Source: CAD feature listing. Evaluate the final solid. Frame: model axes, mm. Face numbers are marked on the shaded views. A direction names the side the tool comes from. Give positions to 0.01 mm unless a question says otherwise; leave off trailing zeros. Order: outer loops, then holes, each group sorted by start corner. A loop starts at its lowest first (then second) coordinate and runs counter-clockwise, first axis right, second up. Notation, with made-up numbers: (11.25, 44.25) - (51.25, 44.25) arc R32 ccw to (51.25, 73.25) - close; hole circle Ø7 at (61.25, -17.75). An arc over 180 degrees is marked (long way). Write each question's results on one line, items separated by ' | '. Start each with the question number.
Item 1: Section C-C on x = 67.5. Output: boundary loops of the cut face in (y, z), and give its area (3 significant figures).
Item 2: Section D-D on x = -80. Output: boundary loops of the cut face in (y, z).
Item 3: Section A-A on z = 45. Output: boundary loops of the cut face in (x, y), and give its area (3 significant figures).
Item 4: Contact query for flat-ended pins moving along their axis: pin 1 Ø4 at (y, z) = (-2.5, 62) entering from +X; pin 2 Ø8.5 at (x, y) = (26.5, 40) entering from +Z; pin 3 Ø8 at (x, y) = (-79.93, 17) entering from +Z; pin 4 Ø12 at (y, z) = (0, 45) entering from -X. Output: stop coordinate, or through.
Item 5: Mould query, pull axis Y, two halves, no side actions, for the marked faces 5, 6, 7 and 8. Classes: released by +Y, released by -Y, zero draft, split by the parting line, or undercut.
Item 6: Set-up query: the marked faces 1, 2, 3 and 4. Return all of +Z, -Z, +X, -X, +Y, -Y with unobstructed straight access to the full face (end or side cutting, diameter ignored); none if empty.
Item 7: Line query: line 1 along Y through (x, z) = (64, 45); line 2 along Y through (x, z) = (-80, 12.5); line 3 along Z through (x, y) = (-58, 9). Output: solid intervals per line, ascending.
Item 8: Section B-B on y = -17. Output: boundary loops of the cut face in (x, z).
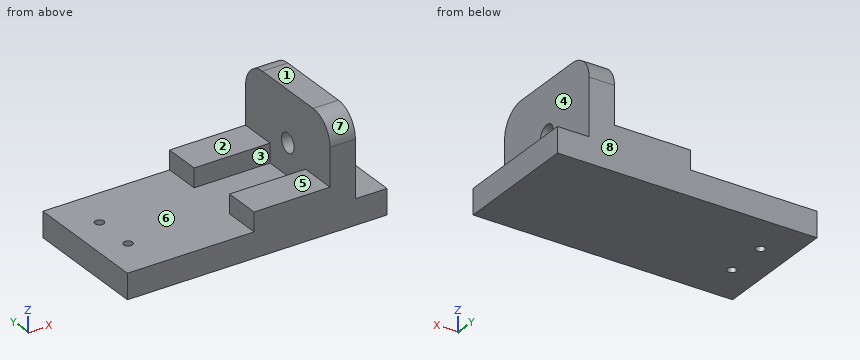
```python
from build123d import *

# Parameters (mm, degrees)
SCHIZZO1_W                   = 205
SCHIZZO1_H                   = 100
ESTRUSIONE_ESTRUSIONE1_DEPTH = 20
FORO_FILETTATO_M8X1_0_1_D    = 7
SCHIZZO6_W                   = 60
SCHIZZO6_H                   = 29
ESTRUSIONE_ESTRUSIONE2_DEPTH = 15
SCHIZZO7_W                   = 20
SCHIZZO7_H                   = 100
ESTRUSIONE_ESTRUSIONE3_DEPTH = 65
SCHIZZO8_R                   = 7.5
TAGLIO_ESTRUSIONE1_DEPTH     = 206.243757518
RACCORDO1_R                  = 20


with BuildPart() as part:
    # Schizzo1 → Estrusione-Estrusione1 (new body)
    with BuildSketch(Plane.XY):
        Rectangle(SCHIZZO1_W, SCHIZZO1_H)
    extrude(amount=ESTRUSIONE_ESTRUSIONE1_DEPTH)

    # Foro filettato M8x1.0-1 (through all)
    with Locations(Plane(origin=(0, 0, 0), x_dir=(-1, 0, 0), z_dir=(0, 0, -1))):
        with Locations((79.93168314, 16.999931365), (80, -17)):
            Hole(FORO_FILETTATO_M8X1_0_1_D / 2)

    # Schizzo6 → Estrusione-Estrusione2 (add)
    with BuildSketch(Plane.XY.offset(20)):
        with Locations((27.5, -35.5)):
            Rectangle(SCHIZZO6_W, SCHIZZO6_H)
        with Locations((27.5, 35.5)):
            Rectangle(SCHIZZO6_W, SCHIZZO6_H)
    extrude(amount=ESTRUSIONE_ESTRUSIONE2_DEPTH)

    # Schizzo7 → Estrusione-Estrusione3 (add)
    with BuildSketch(Plane.XY.offset(20)):
        with Locations((67.5, 0)):
            Rectangle(SCHIZZO7_W, SCHIZZO7_H)
    extrude(amount=ESTRUSIONE_ESTRUSIONE3_DEPTH)

    # Schizzo8 → Taglio-Estrusione1 (cut, through all)
    with BuildSketch(Plane(origin=(77.5, 0, 0), x_dir=(0, 0, -1), z_dir=(1, 0, 0))):
        with Locations((-45, 0)):
            Circle(SCHIZZO8_R)
    extrude(amount=-TAGLIO_ESTRUSIONE1_DEPTH, mode=Mode.SUBTRACT)

    # Raccordo1
    raccordo1_edges = [part.edges().sort_by_distance(p)[0] for p in [
        (67.5, -50, 85),
        (67.5, 50, 85),
    ]]
    fillet(raccordo1_edges, radius=RACCORDO1_R)


solid = part.part
```
Evaluation:
1) outline: (-50, 0) - (50, 0) - (50, 65) arc R20 ccw to (30, 85) - (-30, 85) arc R20 ccw to (-50, 65) - close; hole circle Ø15 at (0, 45) | area: 8,150 mm^2
2) outline: (-50, 0) - (-20.5, 0) - (-20.5, 20) - (-50, 20) - close; (-13.5, 0) - (13.5, 0) - (13.5, 20) - (-13.5, 20) - close; (20.5, 0) - (50, 0) - (50, 20) - (20.5, 20) - close
3) outline: (57.5, -50) - (77.5, -50) - (77.5, -7.5) - (57.5, -7.5) - close; (57.5, 7.5) - (77.5, 7.5) - (77.5, 50) - (57.5, 50) - close | area: 1,700 mm^2
4) pin 1: stops at x = 77.5 | pin 2: stops at z = 35 | pin 3: stops at z = 20 | pin 4: passes through
5) face 5: zero draft | face 6: undercut | face 7: released by -Y | face 8: released by +Y
6) face 1: +Z, +X, -X, +Y, -Y | face 2: +Z, -X, +Y, -Y | face 3: +Z, -X | face 4: +Z, +X, +Y, -Y
7) line 1: y = -50 to -7.5, 7.5 to 50 | line 2: y = -50 to -20.5, -13.5 to 13.5, 20.5 to 50 | line 3: z = 0 to 20
8) outline: (-102.5, 0) - (-83.5, 0) - (-83.5, 20) - (-102.5, 20) - close; (-76.5, 0) - (102.5, 0) - (102.5, 20) - (77.5, 20) - (77.5, 85) - (57.5, 85) - (57.5, 20) - (-76.5, 20) - close
